```python
from build123d import *

# Parameters (mm, degrees)
EXTRUDE_1_DEPTH     = 11.85
SKETCH_2_R          = 1
CUT_EXTRUDE_1_DEPTH = 12.85
FILLET_1_R          = 0.5


with BuildPart() as part:
    # 草图1 → 凸台-拉伸1 (new body)
    with BuildSketch(Plane(origin=(0, 0, 0), x_dir=(1, 0, 0), z_dir=(0, 1, 0))):
        with BuildLine():
            Line((-27.6, 0), (-22.6, 0))
            ThreePointArc((-22.6, 0), (0, 22.6), (22.6, 0))
            Line((22.6, 0), (27.6, 0))
            ThreePointArc((27.6, 0), (0, 27.6), (-27.6, 0))
        make_face()
    extrude(amount=EXTRUDE_1_DEPTH)

    # 草图2 → 切除-拉伸1 (cut, through all)
    with BuildSketch(Plane(origin=(0, 11.85, 0), x_dir=(1, 0, 0), z_dir=(0, 1, 0))):
        with Locations((-25.017738418, 2.03045917)):
            Circle(SKETCH_2_R)
        with Locations((25.017738418, 2.03045917)):
            Circle(SKETCH_2_R)
        with Locations((0, 25.1)):
            Circle(SKETCH_2_R)
    extrude(amount=-CUT_EXTRUDE_1_DEPTH, mode=Mode.SUBTRACT)

    # 圆角1
    fillet_1_edges = [part.edges().sort_by_distance(p)[0] for p in [
        (-22.6, 5.925, 0),
        (-27.6, 5.925, 0),
        (27.6, 5.925, 0),
        (22.6, 5.925, 0),
    ]]
    fillet(fillet_1_edges, radius=FILLET_1_R)


solid = part.part
```
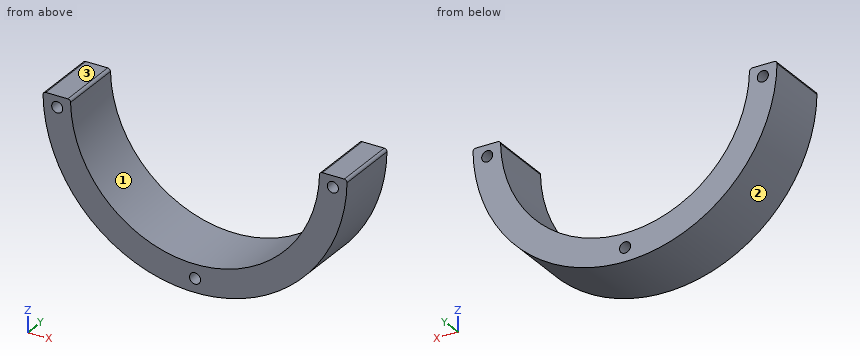
Could you check a few things on this model? Use its own coordinates, in mm. Face numbers are marked on the shaded views. Coordinates: 2 decimals unless noted, no trailing zeros. Loops run counter-clockwise (first coordinate to the right, second up) from the corner with the lowest first, then second, coordinate; pieces in that order, holes last.
1) Imagine slicing it at B-B (z = -25.1). List the corners of the cut face in (x, y) for me, and give its area (3 significant figures).
Reported:
outline: (-11.48, 0) - (-1, 0) - (-1, 11.85) - (-11.48, 11.85) - close; (1, 0) - (11.48, 0) - (11.48, 11.85) - (1, 11.85) - close
area: 248 mm2
2) Will these pins go through, and if not, where does the flat tip stop? pin 1 Ø5 at (x, y) = (15.5, 3.5) entering from +Z; pin 2 Ø1 at (y, z) = (9, -24.5) entering from -X; pin 3 Ø2 at (y, z) = (5, -13) entering from +X; pin 4 Ø1.6 at (x, z) = (25.02, -2.03) entering from -Y.
Reported:
pin 1: stops at z = -13.67
pin 2: stops at x = -13.63
pin 3: stops at x = 24.85
pin 4: passes through
3) Imagine slicing it at D-D (x = -6). List the corners of the cut face in (y, z) for me, and give its area (3 significant figures).
Reported:
outline: (0, -26.94) - (11.85, -26.94) - (11.85, -21.79) - (0, -21.79) - close
area: 61.0 mm2
4) Imagine slicing it at A-A (x = 0). List the corners of the cut face in (y, z) for me, and give its area (4 significant figures).
Reported:
outline: (0, -27.6) - (11.85, -27.6) - (11.85, -26.1) - (0, -26.1) - close; (0, -24.1) - (11.85, -24.1) - (11.85, -22.6) - (0, -22.6) - close
area: 35.55 mm2
5) Please list where these lines run through material, in increasing order: line 1 along X through (y, z) = (6.25, -24.75); line 2 along X through (y, z) = (2, -1); line 3 along X through (y, z) = (7.75, -2.75).
Reported:
line 1: x = -12.21 to -0.94, 0.94 to 12.21
line 2: x = -27.58 to -22.58, 22.58 to 27.58
line 3: x = -27.46 to -25.71, -24.32 to -22.43, 22.43 to 24.32, 25.71 to 27.46
6) Thinking about a two-plate mould opening in X: for the marked faces 1, 2 and 3, which applies, released by +X, released by -X, zero draft, split by the parting line, or undercut?
Reported:
face 1: undercut
face 2: split by the parting line
face 3: zero draft
